Could you check a few things on this model? Use its own coordinates, in mm. A direction names the side the tool comes from. Round coordinates to 2 decimals unless told otherwise and drop trailing zeros. Write each loop counter-clockwise with the first axis right and the second up, starting at its lowest first coordinate (ties: lowest second). Pieces come first, ordered by that corner, then holes. Notation, with made-up numbers: (-37.75, 80.5) -> (-1.75, 80.5) arc R20 cw to (-1.75, 94.5) -> close; hole circle Ø11 at (32, 39). An arc over 180 degrees is marked (long way). One line per question, with ' | ' between items. Start each with the question number.
1. For pin 1 Ø4 at (y, z) = (-29, 25.5) entering from -X; pin 2 Ø16.5 at (x, z) = (-5.5, 12.5) entering from +Y; pin 3 Ø22.5 at (y, z) = (-10.5, 8.5) entering from +X, each with a flat end and sliding along its axis, tell me the tip position at first contact or that it passes through.
2. Imagine slicing it at A-A, the plane z = 29.5. List the corners of the cut face in (x, y) for me.
3. Imagine slicing it at B-B, the plane y = -22.5. List the corners of the cut face in (x, z) for me.
4. Imagine slicing it at D-D, the plane z = 16. List the corners of the cut face in (x, y) for me.
5. If I drill on line 1 along X through (y, z) = (-3, 9.5); line 2 along Y through (x, z) = (8.5, 4); line 3 along Z through (x, y) = (-9, 4.5), over which ranges is the centre line in solid material (lowest first)? Write a range as [from, to].
6. Thinking about a two-plate mould opening in Y: for faces 4 (the flat face through (30.305, -40, 19)), 5 (the flat face through (-36, -41.128, 19)), 6 (the flat face through (34, -36.048, 19)), 7 (the flat face through (32.845, -37, 32)), which applies, released by +Y, released by -Y, zero draft, split by the parting line, or undercut?
7. For faces 1 (the flat face through (-35.755, 14, 32)), 2 (the cylindrical face through (-32.395, -31.555, 4.829)), 3 (the flat face through (-33.215, -40, 19)), which set-ups out of +Z, -Z, +X, -X, +Y, -Y let a thin tool reach every point of the face, with its end or its side?
8. Imagine slicing it at C-C, the plane x = 24.5. List the corners of the cut face in (y, z) for me, and give its area (3 significant figures).
from build123d import *

# Parameters (mm, degrees)
F0_W     = 68.6
F0_H     = 53.4
F1_DEPTH = 25.4
F3_DEPTH = 38.1
F4_DEPTH = 38.1
F7_W     = 59.71
F7_H     = 48.32
F8_DEPTH = 20.32
F9_D     = 2.8448
F9_DEPTH = 9.525
F9_TIP   = 0.8546641445


with BuildPart() as f1:
    # F0 (on Top) → F1 (new body)
    with BuildSketch(Plane.XY):
        with Locations((-1.4553847134, -11.8884605348)):
            Rectangle(F0_W, F0_H)
    extrude(amount=F1_DEPTH)

    # F2 (on face) → F3 (join)
    with BuildSketch(Plane(origin=(0, 0, 0), x_dir=(1, 0, 0), z_dir=(0, 0, -1))):
        Polygon((-35.7553847134, 38.5884605348), (-33.2153847134, 38.5884605348), (-33.2153847134, 41.1284605348), (-38.2953847134, 41.1284605348), (-38.2953847134, 36.0484605348), (-35.7553847134, 36.0484605348), align=None)
    extrude(amount=-F3_DEPTH)

    # F2 (on face) → F4 (join)
    with BuildSketch(Plane(origin=(0, 0, 0), x_dir=(1, 0, 0), z_dir=(0, 0, -1))):
        Polygon((30.3046152866, 41.1284605348), (30.3046152866, 38.5884605348), (32.8446152866, 38.5884605348), (32.8446152866, 36.0484605348), (35.3846152866, 36.0484605348), (35.3846152866, 41.1284605348), align=None)
        Polygon((-35.7553847134, -14.8115394652), (-35.7553847134, -12.2715394652), (-38.2953847134, -12.2715394652), (-38.2953847134, -17.3515394652), (-33.2153847134, -17.3515394652), (-33.2153847134, -14.8115394652), align=None)
        Polygon((35.3846152866, -12.2715394652), (32.8446152866, -12.2715394652), (32.8446152866, -14.8115394652), (30.3046152866, -14.8115394652), (30.3046152866, -17.3515394652), (35.3846152866, -17.3515394652), align=None)
    extrude(amount=-F4_DEPTH)

    # F7 (on Top) → F8 (cut)
    with BuildSketch(Plane.XY):
        with Locations((0.4496152866, -11.8884605348)):
            Rectangle(F7_W, F7_H)
    extrude(amount=F8_DEPTH, mode=Mode.SUBTRACT)

    # F9
    with Locations(Plane(origin=(0, 0, 0), x_dir=(1, 0, 0), z_dir=(0, 0, -1))):
        with Locations((-32.5803847134, 30.1447131348), (-32.5803847134, -6.3677868652)):
            Hole(F9_D / 2, depth=F9_DEPTH)
            with Locations((0, 0, -(F9_DEPTH + F9_TIP / 2))):  # 118° drill point
                Cone(0, F9_D / 2, F9_TIP, mode=Mode.SUBTRACT)


solid = f1.part
Geometry results:
1) pin 1: stops at x = -35.76 | pin 2: stops at y = 14.81 | pin 3: stops at x = 32.84
2) outline: (-38.3, -41.13) -> (-33.22, -41.13) -> (-33.22, -38.59) -> (-35.76, -38.59) -> (-35.76, -36.05) -> (-38.3, -36.05) -> close; (-38.3, 12.27) -> (-35.76, 12.27) -> (-35.76, 14.81) -> (-33.22, 14.81) -> (-33.22, 17.35) -> (-38.3, 17.35) -> close; (30.3, -41.13) -> (35.38, -41.13) -> (35.38, -36.05) -> (32.84, -36.05) -> (32.84, -38.59) -> (30.3, -38.59) -> close; (30.3, 14.81) -> (32.84, 14.81) -> (32.84, 12.27) -> (35.38, 12.27) -> (35.38, 17.35) -> (30.3, 17.35) -> close
3) outline: (-35.76, 0) -> (-29.41, 0) -> (-29.41, 20.32) -> (30.3, 20.32) -> (30.3, 0) -> (32.84, 0) -> (32.84, 25.4) -> (-35.76, 25.4) -> close
4) outline: (-38.3, -41.13) -> (-33.22, -41.13) -> (-33.22, -38.59) -> (30.3, -38.59) -> (30.3, -41.13) -> (35.38, -41.13) -> (35.38, -36.05) -> (32.84, -36.05) -> (32.84, 12.27) -> (35.38, 12.27) -> (35.38, 17.35) -> (30.3, 17.35) -> (30.3, 14.81) -> (-33.22, 14.81) -> (-33.22, 17.35) -> (-38.3, 17.35) -> (-38.3, 12.27) -> (-35.76, 12.27) -> (-35.76, -36.05) -> (-38.3, -36.05) -> close; hole (-29.41, -36.05) -> (30.3, -36.05) -> (30.3, 12.27) -> (-29.41, 12.27) -> close
5) line 1: x = [-35.76, -29.41], [30.3, 32.84] | line 2: y = [-38.59, -36.05], [12.27, 14.81] | line 3: z = [20.32, 25.4]
6) face 4: zero draft | face 5: released by -Y | face 6: undercut | face 7: undercut
7) face 1: +Z | face 2: -Z | face 3: +Z, -Z, -Y
8) outline: (-38.59, 0) -> (-36.05, 0) -> (-36.05, 20.32) -> (12.27, 20.32) -> (12.27, 0) -> (14.81, 0) -> (14.81, 25.4) -> (-38.59, 25.4) -> close | area: 374 mm2
